The listing builds one solid part. Answer for the finished solid, in the listing's coordinates (mm). Face numbers are marked on the shaded views. A direction names the side the tool comes from. Round coordinates to 2 decimals unless told otherwise and drop trailing zeros. Write each loop counter-clockwise with the first axis right and the second up, starting at its lowest first coordinate (ties: lowest second). Pieces come first, ordered by that corner, then holes. Notation, with made-up numbers: (82.25, 17) - (116.25, 17) arc R12 ccw to (116.25, 37) - close; hole circle Ø8 at (-2.5, 89). An arc over 180 degrees is marked (long way). Answer in a Markdown table with one row per item.
from build123d import *

# Parameters (mm, degrees)
F0_R        = 1.5875
F0_R_2      = 17.272
F1_DEPTH    = 2.921
F3_DEPTH    = 20.32
F5_DEPTH    = 16.764
F7_DEPTH    = 55.2085729102
F8_T        = 1.5875
F8_T3_DEPTH = 6.096
F8_T5_DEPTH = 23.495
F8_T7_DEPTH = 25.3893680424
F8_T9_DEPTH = 27.0060511967


# Not quite as in the source:
# - a shell that OpenCascade refuses in one call is made with other operations: the cavity is built on its own and cut out


with BuildPart() as f1:
    # F0 (on Front) → F1 (new body)
    with BuildSketch(Plane.XZ):
        with BuildLine():
            Line((-808.7745012016, 183.0527484417), (-842.3025012016, 183.0527484417))
            Line((-842.3025012016, 183.0527484417), (-842.3025012016, 132.2527484417))
            Line((-842.3025012016, 132.2527484417), (-791.5025012016, 132.2527484417))
            Line((-791.5025012016, 132.2527484417), (-791.5025012016, 165.7807484417))
            ThreePointArc((-791.5025012016, 165.7807484417), (-796.561352877, 177.9938967664), (-808.7745012016, 183.0527484417))
        make_face()
        with Locations((-797.2470434503, 136.9116393686)):
            Circle(F0_R, mode=Mode.SUBTRACT)
        with Locations((-816.9025012016, 157.6527484417)):
            Circle(F0_R_2, mode=Mode.SUBTRACT)
        with Locations((-836.557958953, 178.3938575148)):
            Circle(F0_R, mode=Mode.SUBTRACT)
    extrude(amount=F1_DEPTH)

    # F2 (on face) → F3 (join)
    with BuildSketch(Plane(origin=(-842.3025012016, 0, 0), x_dir=(0, -1, 0), z_dir=(-1, 0, 0))):
        Polygon((2.921, 125.9027484417), (2.921, 132.2527484417), (0, 132.2527484417), (-13.843, 132.2527484417), (-13.843, 125.9027484417), align=None)
    extrude(amount=-F3_DEPTH)

    # F4 (on face) → F5 (join, through all)
    with BuildSketch(Plane.XZ.offset(2.921)):
        with BuildLine():
            Line((-821.9825012016, 125.9027484417), (-842.3025012016, 125.9027484417))
            ThreePointArc((-842.3025012016, 125.9027484417), (-839.0194061041, 113.2468388218), (-829.9981379746, 103.782828939))
            ThreePointArc((-829.9981379746, 103.782828939), (-824.8710634373, 98.8883942721), (-822.1415983833, 92.3468039044))
            ThreePointArc((-822.1415983833, 92.3468039044), (-822.3177482435, 91.6604679901), (-822.9588808932, 91.3587484417))
            Line((-822.9588808932, 91.3587484417), (-833.8504607139, 91.3587484417))
            ThreePointArc((-833.8504607139, 91.3587484417), (-834.438802185, 91.115049425), (-834.6825012016, 90.5267079539))
            Line((-834.6825012016, 90.5267079539), (-834.6825012016, 87.3647889295))
            ThreePointArc((-834.6825012016, 87.3647889295), (-834.438802185, 86.7764474583), (-833.8504607139, 86.5327484417))
            Line((-833.8504607139, 86.5327484417), (-787.9259687792, 86.5327484417))
            ThreePointArc((-787.9259687792, 86.5327484417), (-787.337627308, 86.7764474583), (-787.0939282914, 87.3647889295))
            Line((-787.0939282914, 87.3647889295), (-787.0939282914, 90.5267079539))
            ThreePointArc((-787.0939282914, 90.5267079539), (-787.337627308, 91.115049425), (-787.9259687792, 91.3587484417))
            Line((-787.9259687792, 91.3587484417), (-799.1278296965, 91.3587484417))
            ThreePointArc((-799.1278296965, 91.3587484417), (-799.6417555246, 91.5364406915), (-799.9361712736, 91.9936208083))
            ThreePointArc((-799.9361712736, 91.9936208083), (-803.0180469013, 98.4212453171), (-808.4330915744, 103.0569335505))
            ThreePointArc((-808.4330915744, 103.0569335505), (-818.3403970657, 112.6219563033), (-821.9825012016, 125.9027484417))
        make_face()
    extrude(amount=-F5_DEPTH)

    # F6 (on face) → F7 (cut, through all)
    with BuildSketch(Plane.YZ.offset(-787.0939282914)):
        Polygon((13.843, 91.3587484417), (13.843, 125.9027484417), (5.461, 122.0099536731), (5.461, 91.9936208083), (6.6532706411, 91.3587484417), align=None)
    extrude(amount=-F7_DEPTH, mode=Mode.SUBTRACT)

    # F8: shell of thickness 1.5875, made by hand


with BuildPart() as f8_core1:
    # F8_t2: copy of F1
    add(f1.part)

    # the walls: a layer under each face that stays
    f8_faces = [f8_core1.faces().sort_by_distance(p)[0] for p in [
        (-825.5385012016, -1.4605, 183.0527484417),
        (-814.6982147465, -2.921, 134.7927484417),
        (-838.145458953, -1.4605, 178.3938575148),
        (-834.1745012016, -1.4605, 157.6527484417),
        (-798.8345434503, -1.4605, 136.9116393686),
        (-791.5025012016, -1.4605, 149.0167484417),
        (-806.7425012016, -1.4605, 132.2527484417),
        (-821.9825012016, 5.461, 129.0777484417),
        (-832.1425012016, 13.843, 129.0777484417),
        (-831.9961644541, 9.652, 123.9563510574),
        (-820.9729994901, 5.461, 107.0017872407),
        (-811.0433552949, 6.0571353205, 91.676184625),
        (-812.2898246487, -0.127, 105.6357879061),
        (-803.0180469013, 1.27, 98.4212453171),
        (-799.6417555246, 1.8661353205, 91.5364406915),
        (-787.0939282914, 5.461, 88.9457484417),
        (-810.8882147465, 5.461, 86.5327484417),
        (-834.6825012016, 5.461, 88.9457484417),
        (-795.5800507683, 11.049, 91.3587484417),
        (-822.3177482435, 1.8661353205, 91.6604679901),
        (-824.8710634373, 1.27, 98.8883942721),
        (-841.9306657608, -0.127, 121.5183203365),
        (-833.835834535, 0, 140.7194151084),
        (-842.3025012016, -0.127, 173.5277484417),
        (-796.561352877, -1.4605, 177.9938967664),
    ]]
    thicken(f8_faces, amount=-F8_T, mode=Mode.SUBTRACT)

    # F8_s4 → F8_t3 (cut)
    with BuildSketch(Plane.XZ.offset(-1.5875)):
        Polygon((-821.9666262016, 132.2368734417), (-821.9825012016, 133.8402484417), (-823.5700012016, 133.8402484417), (-823.5700012016, 132.2527484417), align=None)
    extrude(amount=F8_T3_DEPTH, mode=Mode.SUBTRACT)

    # F8_s6 → F8_t5 (cut)
    with BuildSketch(Plane.YZ.offset(-843.5973277066)):
        Polygon((5.4835617697, 121.9955556616), (4.7923230267, 123.4497548244), (3.8735, 123.0230321483), (3.8735, 122.0099536731), align=None)
    extrude(amount=F8_T5_DEPTH, mode=Mode.SUBTRACT)

    # F8_s8 → F8_t7 (cut)
    with BuildSketch(Plane.YZ.offset(-823.7380393161)):
        Polygon((5.4843363881, 92.0076330641), (3.8735, 91.9936208083), (3.8735, 91.0404117704), (4.7148611881, 90.5923952293), align=None)
    extrude(amount=F8_T7_DEPTH, mode=Mode.SUBTRACT)

    # F8_s10 → F8_t9 (cut)
    with BuildSketch(Plane.YZ.offset(-824.5463808932)):
        Polygon((6.6607320292, 91.3886356975), (5.9071318292, 89.9575228626), (6.2569494224, 89.7712484417), (6.6532706411, 89.7712484417), align=None)
    extrude(amount=F8_T9_DEPTH, mode=Mode.SUBTRACT)


with BuildPart() as f1_1:
    add(f1.part)

    # what is left inside the walls is the cavity
    f8_cavity = [f8_core1.part.solids().sort_by_distance(p)[0] for p in [
        (-814.698215, -1.317625, 102.831082),
    ]]
    add(f8_cavity, mode=Mode.SUBTRACT)


solid = f1_1.part
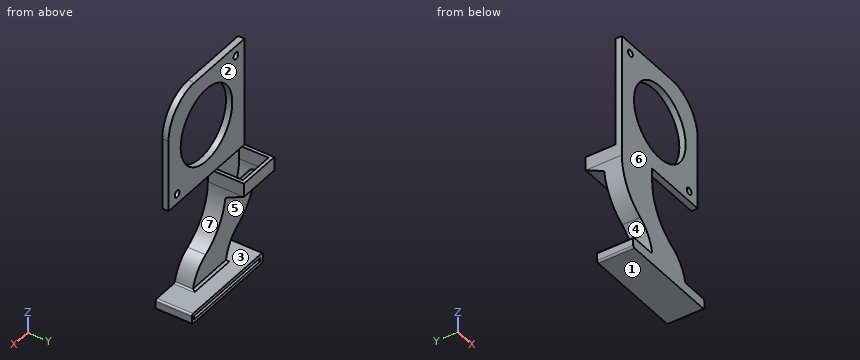
(1) Find the intervals of material crossed by line 1 (Z direction, x = -796.5, y = 13); line 2 (Z direction, x = -824, y = -0.5); line 3 (X direction, y = 6.75, z = 127.5) (1 decimal), in increasing order.
Checked values:
| item | result |
|---|---|
| line 1 | z = 86.53 to 88.12, 89.77 to 91.36 |
| line 2 | z = 86.53 to 88.12, 89.77 to 91.36, 97.48 to 100.4, 132.25 to 141.91, 173.4 to 183.05 |
| line 3 | x = -842.3 to -840.7, -823.6 to -822 |
(2) For the marked faces 4, 5, 6 and 7, determine the directions among +Z, -Z, +X, -X, +Y, -Y from which every point of the face is accessible in a straight line to the end or side of a thin tool.
Checked values:
| item | result |
|---|---|
| face 4 | -X, +Y, -Y |
| face 5 | +X, -X, +Y |
| face 6 | +Z, -Z, +X, -X, -Y |
| face 7 | +X, +Y, -Y |
(3) Section C-C (z = 95.5) is taken. Give the vertices of the cut face in (x, y).
Checked values:
| item | result |
|---|---|
| outline | (-823.06, -2.92) - (-801.21, -2.92) - (-801.21, 5.46) - (-823.06, 5.46) - close; hole (-821.36, -1.33) - (-803, -1.33) - (-803, 3.87) - (-821.36, 3.87) - close |
(4) Section A-A (x = -831.5) is taken. Give the vertices of the cut face in (y, z).
Checked values:
| item | result |
|---|---|
| outline | (-2.92, 86.53) - (13.84, 86.53) - (13.84, 88.12) - (-1.33, 88.12) - (-1.33, 89.77) - (13.84, 89.77) - (13.84, 91.36) - (-2.92, 91.36) - close; (-2.92, 104.79) - (5.46, 104.79) - (5.46, 122.01) - (13.84, 125.9) - (13.84, 132.25) - (12.26, 132.25) - (12.26, 126.92) - (3.87, 123.02) - (3.87, 106.78) - (-1.33, 106.78) - (-1.33, 132.25) - (0, 132.25) - (0, 148.42) - (-2.92, 148.42) - close; (-2.92, 166.89) - (0, 166.89) - (0, 183.05) - (-2.92, 183.05) - close |
(5) For a pull along Z with two mould halves and no side action, classify the marked faces 1, 2 and 3 as pulls with the +Z half, pulls with the -Z half, needs draft (parallel to the pull), parting line crosses it, or undercut.
Checked values:
| item | result |
|---|---|
| face 1 | pulls with the -Z half |
| face 2 | needs draft |
| face 3 | undercut |
(6) Flat-ended cylindrical pins translate along their axes: pin 1 (4 mm diameter, centred on x = -797.25, z = 136.91, fed in from -Y); pin 2 (22 mm diameter, centred on x = -827, z = 110.5, fed in from +Y); pin 3 (7 mm diameter, centred on y = 4, z = 128, fed in from +X); pin 4 (1.5 mm diameter, centred on y = 1, z = 162.5, fed in from -X). Find the tip coordinate at first contact, or state that the pin passes through.
Checked values:
| item | result |
|---|---|
| pin 1 | stops at y = -2.92 |
| pin 2 | stops at y = 5.46 |
| pin 3 | stops at x = -821.94 |
| pin 4 | passes through |
(7) Section B-B (y = 8) is taken. Give the vertices of the cut face in (x, z) (1 decimal).
Checked values:
| item | result |
|---|---|
| outline | (-842.3, 125.9) arc R26 ccw to (-842.2, 123.2) - (-821.8, 123.2) arc R26 cw to (-822, 125.9) - (-822, 132.3) - (-823.6, 132.3) - (-823.6, 125.9) arc R27.6 ccw to (-823.6, 124.9) - (-840.7, 124.9) arc R24.4 cw to (-840.7, 125.9) - (-840.7, 132.3) - (-842.3, 132.3) - close; (-834.7, 87.4) arc R0.8 ccw to (-833.9, 86.5) - (-787.9, 86.5) arc R0.8 ccw to (-787.1, 87.4) - (-787.1, 90.5) arc R0.8 ccw to (-787.9, 91.4) - (-833.9, 91.4) arc R0.8 ccw to (-834.7, 90.5) - close; hole (-833.1, 88.1) - (-788.7, 88.1) - (-788.7, 89.8) - (-833.1, 89.8) - close |
